```python
from build123d import *

# Parameters (mm, degrees)
SKETCH1_W           = 53.5
SKETCH1_H           = 114
SKETCH1_R           = 1.5
SKETCH1_W_2         = 42
SKETCH1_H_2         = 50
BOSS_EXTRUDE1_DEPTH = 3.75
FILLET1_R           = 3
BOSS_EXTRUDE2_DEPTH = 3.75
FILLET2_R           = 1


with BuildPart() as part:
    # Sketch1 → Boss-Extrude1 (new body)
    with BuildSketch(Plane(origin=(0, 0, 0), x_dir=(1, 0, 0), z_dir=(0, 1, 0))):
        with Locations((26.75, 57)):
            Rectangle(SKETCH1_W, SKETCH1_H)
        with Locations(Location((5, 5, 0), (0, 0, 270))):
            Circle(SKETCH1_R, mode=Mode.SUBTRACT)
        with Locations(Location((48.5, 5, 0), (0, 0, 270))):
            Circle(SKETCH1_R, mode=Mode.SUBTRACT)
        with Locations(Location((26.75, 5, 0), (0, 0, 270))):
            Circle(SKETCH1_R, mode=Mode.SUBTRACT)
        with Locations(Location((5, 110, 0), (0, 0, 270))):
            Circle(SKETCH1_R, mode=Mode.SUBTRACT)
        with Locations(Location((48.5, 110, 0), (0, 0, 270))):
            Circle(SKETCH1_R, mode=Mode.SUBTRACT)
        with Locations((26.75, 77)):
            Rectangle(SKETCH1_W_2, SKETCH1_H_2, mode=Mode.SUBTRACT)
    extrude(amount=BOSS_EXTRUDE1_DEPTH)

    # Fillet1
    fillet1_edges = [part.edges().sort_by_distance(p)[0] for p in [
        (5.75, 1.875, -102),
        (5.75, 1.875, -52),
        (47.75, 1.875, -52),
        (47.75, 1.875, -102),
    ]]
    fillet(fillet1_edges, radius=FILLET1_R)

    # Sketch2 → Boss-Extrude2 (add)
    with BuildSketch(Plane(origin=(0, 3.75, 0), x_dir=(1, 0, 0), z_dir=(0, 1, 0))):
        Polygon((0, 114), (-3, 114), (-5, 107), (0, 107), align=None)
        Polygon((53.5, 114), (56.5, 114), (58.5, 107), (53.5, 107), align=None)
    extrude(amount=-BOSS_EXTRUDE2_DEPTH)

    # Fillet2
    fillet2_edges = [part.edges().sort_by_distance(p)[0] for p in [
        (56.5, 1.875, -114),
        (58.5, 1.875, -107),
        (-5, 1.875, -107),
        (-3, 1.875, -114),
    ]]
    fillet(fillet2_edges, radius=FILLET2_R)


solid = part.part
```
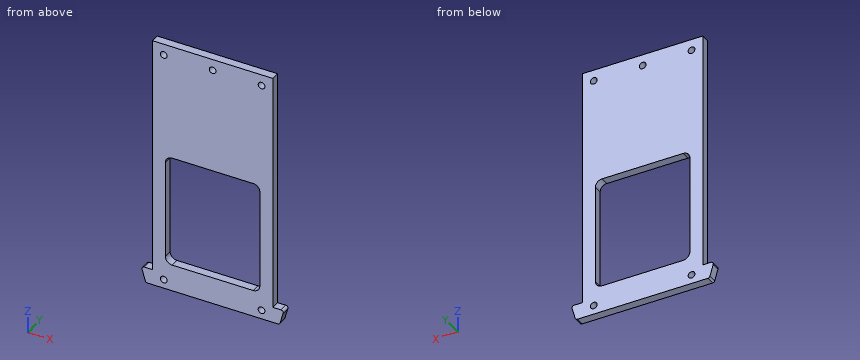
Design review of the part built by this model. Coordinates are the model's own, in mm. Coordinates: 2 decimals unless noted, no trailing zeros. Write each loop counter-clockwise with the first axis right and the second up, starting at its lowest first coordinate (ties: lowest second). Pieces come first, ordered by that corner, then holes.
1) Add section D-D (x = 26.75). Write out the cut boundary in (y, z), plus the area to 3 significant figures.
2) Add section A-A (y = 2.6). Write out the cut boundary in (x, z).
3) To check wall thickness, follow L1, parallel to X at y = 1.25, z = -5; L2, parallel to Z at x = 29, y = 1.15; L3, parallel to X at y = 0.2, z = -57. State the ranges of each line that lie inside material, in increasing order.
4) Add section B-B (x = 13.5). Write out the cut boundary in (y, z), plus the area to 3 significant figures.
5) Add section C-C (z = -66). Write out the cut boundary in (x, y).
6) Insertion check: pin 1 (1.9 mm diameter, centred on y = 2, z = -82.5, fed in from -X); pin 2 (1.1 mm diameter, centred on y = 1, z = -64, fed in from +X). Each pin has a flat end and moves straight along its axis. Give the tip position at first contact, or say it passes through.
Check result:
1. outline: (0, -114) - (3.75, -114) - (3.75, -102) - (0, -102) - close; (0, -52) - (3.75, -52) - (3.75, -6.5) - (0, -6.5) - close; (0, -3.5) - (3.75, -3.5) - (3.75, 0) - (0, 0) - close
1. area: 229 mm2
2. outline: (-4.64, -108.27) - (-3.21, -113.27) arc R1 ccw to (-2.25, -114) - (55.75, -114) arc R1 ccw to (56.71, -113.27) - (58.14, -108.27) arc R1 ccw to (57.17, -107) - (53.5, -107) - (53.5, 0) - (0, 0) - (0, -107) - (-3.67, -107) arc R1 ccw to start; hole circle Ø3 at (5, -110); hole circle Ø3 at (5, -5); hole (5.75, -99) arc R3 ccw to (8.75, -102) - (44.75, -102) arc R3 ccw to (47.75, -99) - (47.75, -55) arc R3 ccw to (44.75, -52) - (8.75, -52) arc R3 ccw to (5.75, -55) - close; hole circle Ø3 at (26.75, -5); hole circle Ø3 at (48.5, -110); hole circle Ø3 at (48.5, -5)
3. L1: x = 0 to 3.5, 6.5 to 25.25, 28.25 to 47, 50 to 53.5
3. L2: z = -114 to -102, -52 to 0
3. L3: x = 0 to 5.75, 47.75 to 53.5
4. outline: (0, -114) - (3.75, -114) - (3.75, -102) - (0, -102) - close; (0, -52) - (3.75, -52) - (3.75, 0) - (0, 0) - close
4. area: 240 mm2
5. outline: (0, 0) - (5.75, 0) - (5.75, 3.75) - (0, 3.75) - close; (47.75, 0) - (53.5, 0) - (53.5, 3.75) - (47.75, 3.75) - close
6. pin 1: stops at x = 0
6. pin 2: stops at x = 53.5
